from build123d import *

# Parameters (mm, degrees)
SKETCH1_W               = 5
SKETCH1_H               = 47
SKETCH2_W               = 18
SKETCH2_H               = 47
BOSS_EXTRUDE1_DEPTH     = 3.5
CUT_EXTRUDE1_DEPTH      = 47
CUT_EXTRUDE1_DEPTH_BACK = 47
SKETCH3_W               = 94
SKETCH3_H               = 94
SKETCH4_W               = 2
SKETCH4_H               = 53.4
CUT_EXTRUDE2_DEPTH      = 23.5
CUT_EXTRUDE2_DEPTH_BACK = 23.5


with BuildPart() as part:
    # Sketch1 → Revolve1 (revolve)
    with BuildSketch(Plane.XY, mode=Mode.PRIVATE) as revolve1_sk:
        with Locations((2.5, 0)):
            Rectangle(SKETCH1_W, SKETCH1_H)
    revolve(revolve1_sk.sketch.rotate(Axis((0, -23.5, 0), (0, 1, 0)), 270), axis=Axis((0, -23.5, 0), (0, 1, 0)))

    # Sketch2 → Boss-Extrude1 (add)
    with BuildSketch(Plane.XY.offset(-5)):
        with Locations((-9, 0)):
            Rectangle(SKETCH2_W, SKETCH2_H)
    extrude(amount=BOSS_EXTRUDE1_DEPTH)

    # Sketch3 → Cut-Extrude1 (cut, two sides: drawn at the far end of the back side and taken through both)
    with BuildSketch(Plane.XY.offset(-CUT_EXTRUDE1_DEPTH_BACK)):
        Rectangle(SKETCH3_W, SKETCH3_H)
        Polygon((-18, -23.5), (-5.25, -23.5), (-5.25, -7.833333333), (5, -7.833333333), (5, 7.833333333), (-5.25, 7.833333333), (-5.25, 23.5), (-18, 23.5), align=None, mode=Mode.SUBTRACT)
    extrude(amount=CUT_EXTRUDE1_DEPTH + CUT_EXTRUDE1_DEPTH_BACK, mode=Mode.SUBTRACT)

    # Sketch4 → Cut-Revolve1 (revolve, cut)
    with BuildSketch(Plane.XY, mode=Mode.PRIVATE) as cut_revolve1_sk:
        with Locations((1, 0)):
            Rectangle(SKETCH4_W, SKETCH4_H)
    revolve(cut_revolve1_sk.sketch.rotate(Axis((0, -26.7, 0), (0, 1, 0)), 270), axis=Axis((0, -26.7, 0), (0, 1, 0)), mode=Mode.SUBTRACT)

    # Sketch5 → Cut-Revolve2 (revolve, cut)
    with BuildSketch(Plane(origin=(-10.5, 0, 0), x_dir=(0, 0, -1), z_dir=(1, 0, 0)), mode=Mode.PRIVATE) as cut_revolve2_sk:
        Polygon((5, -12.5), (5, -15.25), (4.25, -15.25), (1.5, -18), (1.5, -12.5), align=None)
    revolve(cut_revolve2_sk.sketch.rotate(Axis((-10.5, -12.5, -1.5), (0, 0, -1)), 287.341440225), axis=Axis((-10.5, -12.5, -1.5), (0, 0, -1)), mode=Mode.SUBTRACT)

    # Sketch6 → Cut-Revolve3 (revolve, cut)
    with BuildSketch(Plane(origin=(-10.5, 0, 0), x_dir=(0, 0, -1), z_dir=(1, 0, 0)), mode=Mode.PRIVATE) as cut_revolve3_sk:
        Polygon((5, 12.5), (5, 9.75), (4.25, 9.75), (1.5, 7), (1.5, 12.5), align=None)
    revolve(cut_revolve3_sk.sketch.rotate(Axis((-10.5, 12.5, -1.5), (0, 0, -1)), 252.658557197), axis=Axis((-10.5, 12.5, -1.5), (0, 0, -1)), mode=Mode.SUBTRACT)

    # Sketch7 → Cut-Extrude2 (cut, two sides: drawn at the far end of the back side and taken through both)
    with BuildSketch(Plane(origin=(0, 0, 0), x_dir=(1, 0, 0), z_dir=(0, 1, 0)).offset(-CUT_EXTRUDE2_DEPTH_BACK)):
        with BuildLine():
            Line((-18, 1.5), (-17, 1.5))
            ThreePointArc((-17, 1.5), (-17.707106781, 1.792893219), (-18, 2.5))
            Line((-18, 2.5), (-18, 1.5))
        make_face()
    extrude(amount=CUT_EXTRUDE2_DEPTH + CUT_EXTRUDE2_DEPTH_BACK, mode=Mode.SUBTRACT)


solid = part.part
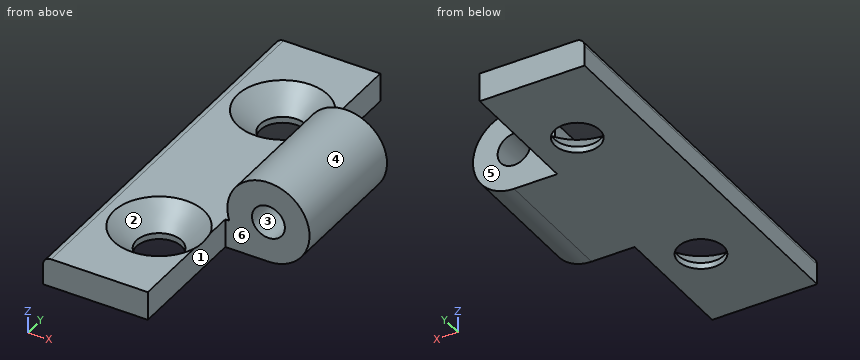
The listing builds one solid part. Answer for the finished solid, in the listing's coordinates (mm). Face numbers are marked on the shaded views. A direction names the side the tool comes from. Coordinates: 2 decimals unless noted, no trailing zeros. Write each loop counter-clockwise with the first axis right and the second up, starting at its lowest first coordinate (ties: lowest second). Pieces come first, ordered by that corner, then holes. Notation, with made-up numbers: M 85,-9.5 L 142,-9.5 A26 ccw 142,8.5 Z; hole C -30,-16 d1. An arc over 180 degrees is marked long. Put each result on its own line as item: value. Start each with the question number.
1. A cutting plane is placed at C-C on y = -12.5. Write down the section's boundary in (x, z).
2. For a pull along Z with two mould halves and no side action, classify the marked faces 1, 2 and 3 as pulls with the +Z half, pulls with the -Z half, needs draft (parallel to the pull), parting line crosses it, or undercut.
3. Which of the six approach directions +Z, -Z, +X, -X, +Y, -Y give full straight-line access (tool end or side, diameter ignored) to the marked faces 4, 5 and 6?
4. A cutting plane is placed at D-D on y = 3.5. Write down the section's boundary in (x, z), then the cut area to 3 significant figures.
5. Flat-ended cylindrical pins translate along their axes: P1, Ø5, axis at x = 0, z = -1.5, coming from the -Y side; P2, Ø1, axis at y = -17.5, z = -2.5, coming from the +X side; P3, Ø1, axis at y = -8, z = 3, coming from the -X side. Find the tip coordinate at first contact, or state that the pin passes through.
6. A cutting plane is placed at A-A on z = 0. Write down the section's boundary in (x, y).
7. Consider line 1 (Y direction, x = -10.5, z = -4.5); line 2 (X direction, y = -1.75, z = 0); line 3 (X direction, y = 12.5, z = -4.6). Determine where each line is inside the solid, lowest interval first. Write a range as from..to.
8. A cutting plane is placed at B-B on x = -10.5. Write down the section's boundary in (y, z).
Resolved:
1. outline: M -18,-5 L -13.25,-5 L -13.25,-4.25 L -16,-1.5 L -17,-1.5 A1 ccw -18,-2.5 Z; M -7.75,-5 L -5.25,-5 L -5.25,-1.75 L -7.75,-4.25 Z
2. face 1: needs draft
2. face 2: pulls with the +Z half
2. face 3: undercut
3. face 4: +Y, -Y
3. face 5: +Z, -Z, +X, +Y
3. face 6: +Z, -Z, +X, -Y
4. outline: M -18,-5 L 0,-5 A5 ccw long -4.77,-1.5 L -17,-1.5 A1 ccw -18,-2.5 Z; hole C 0,0 d4
4. area: 117 mm2
5. P1: stops at y = -7.83
5. P2: stops at x = -5.25
5. P3: stops at x = -4.31
6. outline: M -5,-7.83 L -2,-7.83 L -2,7.83 L -5,7.83 Z; M 2,-7.83 L 5,-7.83 L 5,7.83 L 2,7.83 Z
7. line 1: y = -23.5..-15.25, -9.75..9.75, 15.25..23.5
7. line 2: x = -5..-2, 2..5
7. line 3: x = -18..-13.25, -7.75..-5.25
8. outline: M -23.5,-5 L -15.25,-5 L -15.25,-4.25 L -18,-1.5 L -23.5,-1.5 Z; M -9.75,-5 L 9.75,-5 L 9.75,-4.25 L 7,-1.5 L -7,-1.5 L -9.75,-4.25 Z; M 15.25,-5 L 23.5,-5 L 23.5,-1.5 L 18,-1.5 L 15.25,-4.25 Z
